```python
from build123d import *

# Parameters (mm, degrees)
SKETCH1_W           = 35
SKETCH1_H           = 30
SKETCH1_W_2         = 2.5
SKETCH1_H_2         = 9
BOSS_EXTRUDE1_DEPTH = 4.5
FILLET1_R           = 5
SKETCH2_W           = 4.5
SKETCH2_H           = 15
CUT_EXTRUDE1_DEPTH  = 4.5


with BuildPart() as part:
    # Sketch1 → Boss-Extrude1 (new body)
    with BuildSketch(Plane.XY):
        Rectangle(SKETCH1_W, SKETCH1_H)
        with Locations((-16.25, -19.5)):
            Rectangle(SKETCH1_W_2, SKETCH1_H_2)
        with Locations((16.25, -19.5)):
            Rectangle(SKETCH1_W_2, SKETCH1_H_2)
    extrude(amount=BOSS_EXTRUDE1_DEPTH)

    # Fillet1
    fillet1_edges = [part.edges().sort_by_distance(p)[0] for p in [
        (-17.5, 15, 2.25),
        (17.5, 15, 2.25),
    ]]
    fillet(fillet1_edges, radius=FILLET1_R)

    # Sketch2 → Cut-Extrude1 (cut)
    with BuildSketch(Plane.XY.offset(4.5)):
        with Locations((0, 7.5)):
            Rectangle(SKETCH2_W, SKETCH2_H)
    extrude(amount=-CUT_EXTRUDE1_DEPTH, mode=Mode.SUBTRACT)


solid = part.part
```
CAD build for the part. Positions are in the model's coordinates, mm. A direction names the side the tool comes from. Round coordinates to 2 decimals unless told otherwise and drop trailing zeros. Write each loop counter-clockwise with the first axis right and the second up, starting at its lowest first coordinate (ties: lowest second). Pieces come first, ordered by that corner, then holes. Notation, with made-up numbers: (74.5, 42) - (80.5, 42) arc R27 cw to (80.5, 71) - close; hole circle Ø9 at (14, 35.25). An arc over 180 degrees is marked (long way). Return JSON: item names as keys, results as strings. Group by question number.
Item 1: Probe probe 1 along X at (y, z) = (1, 2.65); probe 2 along X at (y, z) = (-17, 0.65); probe 3 along Y at (x, z) = (-5, 1.15). List the from-to ranges inside material, lowest first.
Item 2: Band-saw the part on C-C on x = 0. List the corners of the cut face in (y, z).
Item 3: Flat gauge pins, fed straight in: pin 1 Ø1.5 at (x, z) = (0.5, 2.5) entering from +Y; pin 2 Ø1.5 at (x, z) = (5.5, 2.5) entering from -Y. Where does each tip first touch, or does it go through?
Item 4: Band-saw the part on B-B on z = 3.4. List the corners of the cut face in (x, y), plus the area to 3 significant figures.
Item 5: Band-saw the part on D-D on y = -16. List the corners of the cut face in (x, z).
Item 6: Mould opens along X. For faces 4 (the face through (15, -20, 2)), 5 (the face through (-17.5, -7, 2)), 6 (the face through (7, 15, 2)) say: +X half, -X half, draft (parallel to the pull), parting line (faces both ways), or undercut.
Item 7: 3-axis set-ups, long thin cutter, end or side, ignore diameter. For faces 1 (the face through (-15, -20, 2)), 2 (the face through (0, -4, 4.5)), 3 (the face through (0, 0, 2)): which of +Z, -Z, +X, -X, +Y, -Y reach the whole face in a straight line?
Item 8: Band-saw the part on A-A on y = 2. List the corners of the cut face in (x, z).
Resolved:
{
 "1": {"probe 1": "x = -17.5 to -2.25, 2.25 to 17.5", "probe 2": "x = -17.5 to -15, 15 to 17.5", "probe 3": "y = -15 to 15"},
 "2": {"outline": "(-15, 0) - (0, 0) - (0, 4.5) - (-15, 4.5) - close"},
 "3": {"pin 1": "stops at y = 0", "pin 2": "stops at y = -15"},
 "4": {"outline": "(-17.5, -24) - (-15, -24) - (-15, -15) - (15, -15) - (15, -24) - (17.5, -24) - (17.5, 10) arc R5 ccw to (12.5, 15) - (2.25, 15) - (2.25, 0) - (-2.25, 0) - (-2.25, 15) - (-12.5, 15) arc R5 ccw to (-17.5, 10) - close", "area": "1,020 mm²"},
 "5": {"outline": "(-17.5, 0) - (-15, 0) - (-15, 4.5) - (-17.5, 4.5) - close; (15, 0) - (17.5, 0) - (17.5, 4.5) - (15, 4.5) - close"},
 "6": {"face 4": "undercut", "face 5": "-X half", "face 6": "draft"},
 "7": {"face 1": "+Z, -Z, -Y", "face 2": "+Z, +X, -X, +Y, -Y", "face 3": "+Z, -Z, +Y"},
 "8": {"outline": "(-17.5, 0) - (-2.25, 0) - (-2.25, 4.5) - (-17.5, 4.5) - close; (2.25, 0) - (17.5, 0) - (17.5, 4.5) - (2.25, 4.5) - close"}
}
